from build123d import *

# Parameters (mm, degrees)
SKETCH046_W   = 70
SKETCH046_H   = 160
SKETCH046_R   = 2.8
SKETCH046_R_2 = 6.15
SKETCH046_R_3 = 7.15
PAD021_DEPTH  = 3
SKETCH047_W   = 65
SKETCH047_H   = 140
SKETCH047_W_2 = 62
SKETCH047_H_2 = 137
PAD022_DEPTH  = 7
FILLET018_R   = 1
FILLET019_R   = 5
FILLET020_R   = 2


with BuildPart() as part:
    # Sketch046 → Pad021 (new body)
    with BuildSketch(Plane.XY):
        Rectangle(SKETCH046_W, SKETCH046_H)
        with Locations((-29, 75)):
            Circle(SKETCH046_R, mode=Mode.SUBTRACT)
        with Locations((29, 75)):
            Circle(SKETCH046_R, mode=Mode.SUBTRACT)
        with Locations((-29, -75)):
            Circle(SKETCH046_R, mode=Mode.SUBTRACT)
        with Locations((29, -75)):
            Circle(SKETCH046_R, mode=Mode.SUBTRACT)
        with Locations((0, -60)):
            Circle(SKETCH046_R_2, mode=Mode.SUBTRACT)
        with Locations((0, -20)):
            Circle(SKETCH046_R_2, mode=Mode.SUBTRACT)
        with Locations((0, -40)):
            Circle(SKETCH046_R_3, mode=Mode.SUBTRACT)
        with Locations((20, -40)):
            Circle(SKETCH046_R_2, mode=Mode.SUBTRACT)
        with Locations((-20, -40)):
            Circle(SKETCH046_R_2, mode=Mode.SUBTRACT)
        with Locations((-16, 58)):
            Circle(SKETCH046_R_2, mode=Mode.SUBTRACT)
        with Locations((16, 58)):
            Circle(SKETCH046_R_2, mode=Mode.SUBTRACT)
        with Locations((-16, 31)):
            Circle(SKETCH046_R_2, mode=Mode.SUBTRACT)
        with Locations((16, 31)):
            Circle(SKETCH046_R_2, mode=Mode.SUBTRACT)
        with Locations((-16, 4)):
            Circle(SKETCH046_R_2, mode=Mode.SUBTRACT)
        with Locations((16, 4)):
            Circle(SKETCH046_R_2, mode=Mode.SUBTRACT)
    extrude(amount=PAD021_DEPTH)

    # Sketch047 (on Face20 of Pad021) → Pad022 (join)
    with BuildSketch(Plane(origin=(0, 0, 0), x_dir=(1, 0, 0), z_dir=(0, 0, -1))):
        Rectangle(SKETCH047_W, SKETCH047_H)
        Rectangle(SKETCH047_W_2, SKETCH047_H_2, mode=Mode.SUBTRACT)
    extrude(amount=PAD022_DEPTH)

    # Fillet018
    fillet018_edges = [part.edges().sort_by_distance(p)[0] for p in [
        (0, 68.5, 0),
        (31, 0, 0),
        (-31, 0, 0),
        (0, -68.5, 0),
    ]]
    fillet(fillet018_edges, radius=FILLET018_R)

    # Fillet019
    fillet019_edges = [part.edges().sort_by_distance(p)[0] for p in [
        (-35, 80, 1.5),
        (35, 80, 1.5),
        (-35, -80, 1.5),
        (35, -80, 1.5),
    ]]
    fillet(fillet019_edges, radius=FILLET019_R)

    # Fillet020
    fillet020_edges = [part.edges().sort_by_distance(p)[0] for p in [
        (-32.5, -70, -3.5),
        (32.5, -70, -3.5),
        (-32.5, 70, -3.5),
        (32.5, 70, -3.5),
    ]]
    fillet(fillet020_edges, radius=FILLET020_R)


solid = part.part
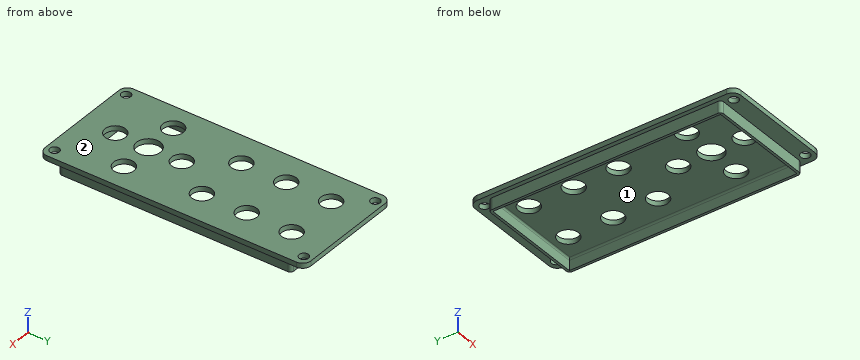
Verification items for the finished model (mm, model axes). Face numbers are marked on the shaded views. Round coordinates to 2 decimals unless told otherwise and drop trailing zeros. Order: outer loops, then holes, each group sorted by start corner. A loop starts at its lowest first (then second) coordinate and runs counter-clockwise, first axis right, second up. Notation, with made-up numbers: (26.5, 71) -> (35.5, 71) arc R25 cw to (35.5, 109) -> close; hole circle Ø6 at (87.25, 31). An arc over 180 degrees is marked (long way). Put each result on its own line as item: value.
1) Material ranges on line 1 (Y direction, x = 0, z = 1.75); line 2 (X direction, y = 13, z = -1.75); line 3 (Y direction, x = -6.5, z = -2.75), recorded low to high.
Final values:
line 1: y = -80 to -66.15, -53.85 to -47.15, -32.85 to -26.15, -13.85 to 80
line 2: x = -32.5 to -31, 31 to 32.5
line 3: y = -70 to -68.5, 68.5 to 70
2) Section check C-C (y = -60). Record the cut outline in (x, z), then the cut area to 3 significant figures.
Final values:
outline: (-35, 0) -> (-32.5, 0) -> (-32.5, -7) -> (-31, -7) -> (-31, -1) arc R1 cw to (-30, 0) -> (-6.15, 0) -> (-6.15, 3) -> (-35, 3) -> close; (6.15, 0) -> (30, 0) arc R1 cw to (31, -1) -> (31, -7) -> (32.5, -7) -> (32.5, 0) -> (35, 0) -> (35, 3) -> (6.15, 3) -> close
area: 195 mm^2
3) Mould release check, pull along X, two halves, no side actions. Record for the marked faces 1 and 2: +X half, -X half, draft (parallel to the pull), parting line (faces both ways), or undercut.
Final values:
face 1: undercut
face 2: draft
4) Section check D-D (x = -16). Give the number of separate pieces and of enclosed holes in the cut face, then the cut area to 3 significant figures.
Final values:
separate pieces: 5
enclosed holes: 0
area: 363 mm^2
5) Section check B-B (y = 58). Record the cut outline in (x, z).
Final values:
outline: (-35, 0) -> (-32.5, 0) -> (-32.5, -7) -> (-31, -7) -> (-31, -1) arc R1 cw to (-30, 0) -> (-22.15, 0) -> (-22.15, 3) -> (-35, 3) -> close; (-9.85, 0) -> (9.85, 0) -> (9.85, 3) -> (-9.85, 3) -> close; (22.15, 0) -> (30, 0) arc R1 cw to (31, -1) -> (31, -7) -> (32.5, -7) -> (32.5, 0) -> (35, 0) -> (35, 3) -> (22.15, 3) -> close
6) Section check A-A (z = -4.5). Record the cut outline in (x, y), then the cut area to 3 significant figures.
Final values:
outline: (-32.5, -68) arc R2 ccw to (-30.5, -70) -> (30.5, -70) arc R2 ccw to (32.5, -68) -> (32.5, 68) arc R2 ccw to (30.5, 70) -> (-30.5, 70) arc R2 ccw to (-32.5, 68) -> close; hole (-31, -68.5) -> (31, -68.5) -> (31, 68.5) -> (-31, 68.5) -> close
area: 603 mm^2
7) Depth check by flat-ended pin: pin 1 (16 mm diameter, centred on x = 16, y = 58, fed in from -Z); pin 2 (3.5 mm diameter, centred on y = 22, z = -2.5, fed in from +X); pin 3 (3.5 mm diameter, centred on x = -9.5, z = -4, fed in from -Y); pin 4 (5 mm diameter, centred on x = -29, y = 75, fed in from -Z). Enter the tip coordinate at first touch or a pass-through.
Final values:
pin 1: stops at z = 0
pin 2: stops at x = 32.5
pin 3: stops at y = -70
pin 4: passes through
